Could you check a few things on this model? Use its own coordinates, in mm. Face numbers are marked on the shaded views. A direction names the side the tool comes from. Give positions to 0.01 mm unless a question says otherwise; leave off trailing zeros. Order: outer loops, then holes, each group sorted by start corner. A loop starts at its lowest first (then second) coordinate and runs counter-clockwise, first axis right, second up. Notation, with made-up numbers: M -21,14.5 L 33,14.5 A20 ccw 33,53.5 Z; hole C -12.75,48 d8. An arc over 180 degrees is marked long. Return JSON: item names as keys, results as strings. Group by question number.
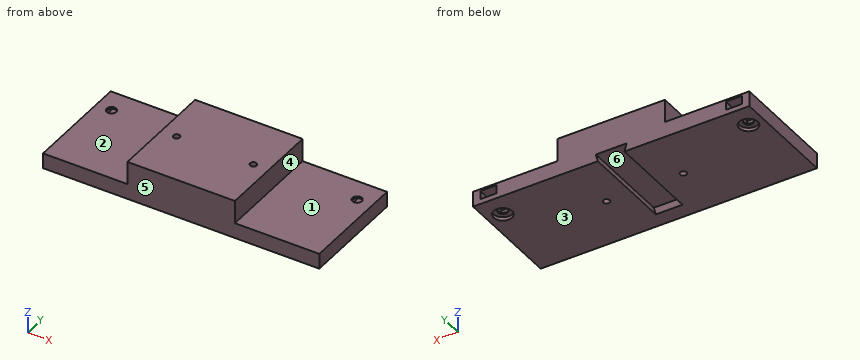
```python
from build123d import *

# Parameters (mm, degrees)
SKIZZE1_W                       = 180
SKIZZE1_H                       = 70
SKIZZE1_R                       = 2.1
SKIZZE1_R_2                     = 3.1
AUFSATZ_LINEAR_AUSTRAGEN2_DEPTH = 25
SKIZZE4_W                       = 55
SKIZZE4_H                       = 70
SCHNITT_LINEAR_AUSTRAGEN1_DEPTH = 15
SKIZZE5_W                       = 10.5
SKIZZE5_H                       = 5.5
SCHNITT_LINEAR_AUSTRAGEN2_DEPTH = 22
SKIZZE6_R                       = 6
SCHNITT_LINEAR_AUSTRAGEN3_DEPTH = 2.3
SCHNITT_LINEAR_AUSTRAGEN4_DEPTH = 60


with BuildPart() as part:
    # Skizze1 → Aufsatz-Linear austragen2 (new body)
    with BuildSketch(Plane.XY):
        Rectangle(SKIZZE1_W, SKIZZE1_H)
        with Locations((25, 0)):
            Circle(SKIZZE1_R, mode=Mode.SUBTRACT)
        with Locations(Location((-25, 0, 0), (0, 0, 180))):
            Circle(SKIZZE1_R, mode=Mode.SUBTRACT)
        with Locations((80, 20)):
            Circle(SKIZZE1_R_2, mode=Mode.SUBTRACT)
        with Locations(Location((-80, 20, 0), (0, 0, 180))):
            Circle(SKIZZE1_R_2, mode=Mode.SUBTRACT)
    extrude(amount=AUFSATZ_LINEAR_AUSTRAGEN2_DEPTH)

    # Skizze4 → Schnitt-Linear austragen1 (cut)
    with BuildSketch(Plane.XY.offset(25)):
        with Locations((62.5, 0)):
            Rectangle(SKIZZE4_W, SKIZZE4_H)
        with Locations((-62.5, 0)):
            Rectangle(SKIZZE4_W, SKIZZE4_H)
    extrude(amount=-SCHNITT_LINEAR_AUSTRAGEN1_DEPTH, mode=Mode.SUBTRACT)

    # Skizze5 → Schnitt-Linear austragen2 (cut)
    with BuildSketch(Plane(origin=(0, 35, 0), x_dir=(1, 0, 0), z_dir=(0, 1, 0))):
        with Locations((80, -6)):
            Rectangle(SKIZZE5_W, SKIZZE5_H)
        with Locations((-80, -6)):
            Rectangle(SKIZZE5_W, SKIZZE5_H)
    extrude(amount=-SCHNITT_LINEAR_AUSTRAGEN2_DEPTH, mode=Mode.SUBTRACT)

    # Skizze6 → Schnitt-Linear austragen3 (cut)
    with BuildSketch(Plane(origin=(0, 0, 0), x_dir=(-1, 0, 0), z_dir=(0, 0, -1))):
        with Locations((-80, 20)):
            Circle(SKIZZE6_R)
        with Locations(Location((80, 20, 0), (0, 0, 180))):
            Circle(SKIZZE6_R)
    extrude(amount=-SCHNITT_LINEAR_AUSTRAGEN3_DEPTH, mode=Mode.SUBTRACT)

    # Skizze7 → Schnitt-Linear austragen4 (cut)
    with BuildSketch(Plane(origin=(0, 35, 0), x_dir=(1, 0, 0), z_dir=(0, 1, 0))):
        Polygon((8.660254038, 0), (-8.660254038, 0), (-10, -5), (10, -5), align=None)
    extrude(amount=-SCHNITT_LINEAR_AUSTRAGEN4_DEPTH, mode=Mode.SUBTRACT)


solid = part.part
```
1. Imagine slicing it at A-A, the plane y = 0. Please give me the cut outline in (x, z), plus the area to 3 significant figures.
2. Imagine slicing it at B-B, the plane x = 80. Please give me the cut outline in (y, z), plus the area to 3 significant figures.
3. Imagine slicing it at D-D, the plane x = 25. Please give me the cut outline in (y, z).
4. If we mould it in two halves opening along X, with no side actions, what happens to the marked faces 4, 5 and 6? For each: pulls with the +X half, pulls with the -X half, needs draft (parallel to the pull), parting line crosses it, or undercut.
5. I need wall thicknesses on L1, parallel to Y at x = 80, z = 1.3; L2, parallel to Y at x = -80, z = 2.65; L3, parallel to X at y = 1, z = 20. Which ranges of each line are inside material? Lowest first, please. Write a range as from..to.
6. Which directions (+Z, -Z, +X, -X, +Y, -Y) give clear straight access to the entire face, cutting with the end or side of a thin tool? Please do the marked faces 1, 2 and 3.
7. Imagine slicing it at C-C, the plane z = 13.75. Please give me the cut outline in (x, y).
8. For pin 1 (8 mm diameter, centred on y = 15, z = 19.5, fed in from +X); pin 2 (4.5 mm diameter, centred on x = 81.5, z = 7, fed in from +Y); pin 3 (3.5 mm diameter, centred on x = 77.5, y = 18, fed in from -Z); pin 4 (5.5 mm diameter, centred on x = 80, y = 20, fed in from -Z), each with a flat end and sliding along its axis, tell me the tip position at first contact or that it passes through.
Values:
{
 "1": {"outline": "M -90,0 L -27.1,0 L -27.1,25 L -35,25 L -35,10 L -90,10 Z; M -22.9,0 L -8.66,0 L -10,5 L 10,5 L 8.66,0 L 22.9,0 L 22.9,25 L -22.9,25 Z; M 27.1,0 L 90,0 L 90,10 L 35,10 L 35,25 L 27.1,25 Z", "area": "2,550 mm²"},
 "2": {"outline": "M -35,0 L 14,0 L 14,2.3 L 16.9,2.3 L 16.9,3.25 L 13,3.25 L 13,8.75 L 16.9,8.75 L 16.9,10 L -35,10 Z; M 23.1,2.3 L 26,2.3 L 26,0 L 35,0 L 35,3.25 L 23.1,3.25 Z; M 23.1,8.75 L 35,8.75 L 35,10 L 23.1,10 Z", "area": "538 mm²"},
 "3": {"outline": "M -35,0 L -2.1,0 L -2.1,25 L -35,25 Z; M 2.1,0 L 35,0 L 35,25 L 2.1,25 Z"},
 "4": {"face 4": "pulls with the +X half", "face 5": "needs draft", "face 6": "undercut"},
 "5": {"L1": "y = -35..14, 26..35", "L2": "y = -35..16.9, 23.1..35", "L3": "x = -35..-26.85, -23.15..23.15, 26.85..35"},
 "6": {"face 1": "+Z, +X, +Y, -Y", "face 2": "+Z, -X, +Y, -Y", "face 3": "-Z, +X, -X, +Y, -Y"},
 "7": {"outline": "M -35,-35 L 35,-35 L 35,35 L -35,35 Z; hole C -25,0 d4.2; hole C 25,0 d4.2"},
 "8": {"pin 1": "stops at x = 35", "pin 2": "stops at y = 35", "pin 3": "stops at z = 2.3", "pin 4": "passes through"}
}
